CAD build for the part. Positions are in the model's coordinates, mm. Give positions to 0.01 mm unless a question says otherwise; leave off trailing zeros. Write each loop counter-clockwise with the first axis right and the second up, starting at its lowest first coordinate (ties: lowest second). Pieces come first, ordered by that corner, then holes. Notation, with made-up numbers: (68.25, 11) - (121.25, 11) arc R5 cw to (121.25, 16) - close; hole circle Ø10 at (-6.5, -4). An arc over 180 degrees is marked (long way). Put each result on its own line as item: value. Start each with the question number.
1. Cut at A-A on x = 9.5. List the corners of the cut face in (y, z).
2. Cut at B-B on z = 0. List the corners of the cut face in (x, y), and give its area (3 significant figures).
3. Drop flat-ended pins along their axis: pin 1 (0.8 mm diameter, centred on y = -3.5, z = -2, fed in from -X); pin 2 (2.5 mm diameter, centred on y = -1.5, z = -0.5, fed in from +X). Give the stop position or say it passes through.
4. Wall check: line 1 (Z direction, x = -1.5, y = -4.7); line 2 (Z direction, x = 40, y = -2.95); line 3 (X direction, y = -1, z = -6.5). Give the ranges that are in metal, low to high.
from build123d import *

# Parameters (mm, degrees)
F1_DEPTH = 5


with BuildPart() as f1:
    # F0 (on Front) → F1 (new body)
    with BuildSketch(Plane.XZ):
        Polygon((-58.772724, -16), (0, -16), (58.772724, -16), (58.772724, -6), (43.212797, -6), (43.212797, -1.5), (37.212797, -1.5), (37.212797, -2.5), (34.212797, -2.5), (34.212797, -1.5), (31.168662, -1.5), (31.168662, 0), (31.168662, 1.5), (34.212797, 1.5), (34.212797, 2.5), (37.212797, 2.5), (37.212797, 1.5), (43.212797, 1.5), (43.212797, 6), (58.772724, 6), (58.772724, 16), (0, 16), (-58.772724, 16), (-58.772724, 6), (-43.212797, 6), (-43.212797, 1.5), (-37.212797, 1.5), (-37.212797, 2.5), (-34.212797, 2.5), (-34.212797, 1.5), (-31.168662, 1.5), (-31.168662, 0), (-31.168662, -1.5), (-34.212797, -1.5), (-34.212797, -2.5), (-37.212797, -2.5), (-37.212797, -1.5), (-43.212797, -1.5), (-43.212797, -6), (-58.772724, -6), align=None)
        with BuildLine():
            ThreePointArc((12.272724, 7.5), (19.772724, 0), (12.272724, -7.5))
            Line((12.272724, -7.5), (0, -7.5))
            Line((0, -7.5), (-12.272724, -7.5))
            ThreePointArc((-12.272724, -7.5), (-19.772724, 0), (-12.272724, 7.5))
            Line((-12.272724, 7.5), (0, 7.5))
            Line((0, 7.5), (12.272724, 7.5))
        make_face(mode=Mode.SUBTRACT)
    extrude(amount=F1_DEPTH)


solid = f1.part
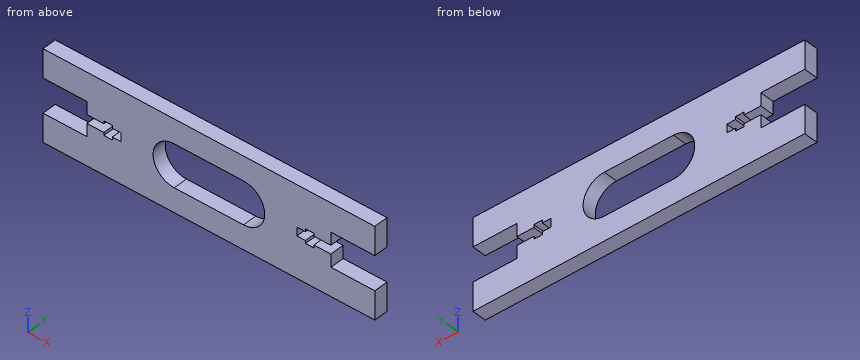
Report:
1. outline: (-5, -16) - (0, -16) - (0, -7.5) - (-5, -7.5) - close; (-5, 7.5) - (0, 7.5) - (0, 16) - (-5, 16) - close
2. outline: (-31.17, -5) - (-19.77, -5) - (-19.77, 0) - (-31.17, 0) - close; (19.77, -5) - (31.17, -5) - (31.17, 0) - (19.77, 0) - close
2. area: 114 mm²
3. pin 1: stops at x = -43.21
3. pin 2: stops at x = 43.21
4. line 1: z = -16 to -7.5, 7.5 to 16
4. line 2: z = -16 to -1.5, 1.5 to 16
4. line 3: x = -58.77 to -16.01, 16.01 to 58.77
